Source: CAD feature listing. Evaluate the final solid. Frame: model axes, mm. Face numbers are marked on the shaded views. A direction names the side the tool comes from. Round coordinates to 2 decimals unless told otherwise and drop trailing zeros. Order: outer loops, then holes, each group sorted by start corner. A loop starts at its lowest first (then second) coordinate and runs counter-clockwise, first axis right, second up. Notation, with made-up numbers: (81, 83.25) -> (129, 83.25) arc R29 cw to (129, 110.25) -> close; hole circle Ø6 at (-18.75, 39). An arc over 180 degrees is marked (long way). Answer as CSV lines item,"result".
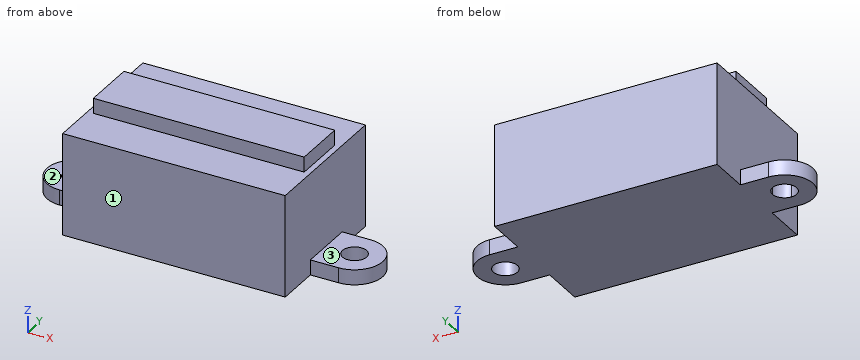
from build123d import *

# Parameters (mm, degrees)
F0_W     = 29.5
F0_H     = 18.9
F1_DEPTH = 13.5
F2_R     = 1.6
F3_DEPTH = 2
F4_W     = 27.95
F4_H     = 7.2
F5_DEPTH = 2


with BuildPart() as f1:
    # F0 (on Top) → F1 (new body)
    with BuildSketch(Plane.XY):
        with Locations((-2.3268059269, -8.9522809724)):
            Rectangle(F0_W, F0_H)
    extrude(amount=F1_DEPTH)

    # F2 (on face) → F3 (join)
    with BuildSketch(Plane(origin=(0, 0, 0), x_dir=(1, 0, 0), z_dir=(0, 0, -1))):
        with BuildLine():
            Line((-20.8268059269, 7.1262256302), (-20.8268059269, 4.9762256302))
            Line((-20.8268059269, 4.9762256302), (-17.0768059269, 4.9762256302))
            Line((-17.0768059269, 4.9762256302), (-17.0768059269, 12.4762256302))
            Line((-17.0768059269, 12.4762256302), (-20.8268059269, 12.4762256302))
            Line((-20.8268059269, 12.4762256302), (-20.8268059269, 10.3262256302))
            ThreePointArc((-20.8268059269, 10.3262256302), (-19.695435077, 9.8575964801), (-19.2268059269, 8.7262256302))
            ThreePointArc((-19.2268059269, 8.7262256302), (-19.695435077, 7.5948547803), (-20.8268059269, 7.1262256302))
        make_face()
        with BuildLine():
            ThreePointArc((-20.8268059269, 12.4762256302), (-24.5768059269, 8.7262256302), (-20.8268059269, 4.9762256302))
            Line((-20.8268059269, 4.9762256302), (-20.8268059269, 7.1262256302))
            ThreePointArc((-20.8268059269, 7.1262256302), (-22.4268059269, 8.7262256302), (-20.8268059269, 10.3262256302))
            Line((-20.8268059269, 10.3262256302), (-20.8268059269, 12.4762256302))
        make_face()
        with BuildLine():
            Line((12.4231940731, 12.4762256302), (12.4231940731, 4.9762256302))
            Line((12.4231940731, 4.9762256302), (16.1731940731, 4.9762256302))
            ThreePointArc((16.1731940731, 4.9762256302), (19.9231940731, 8.7262256302), (16.1731940731, 12.4762256302))
            Line((16.1731940731, 12.4762256302), (12.4231940731, 12.4762256302))
        make_face()
        with Locations((16.1731940731, 8.7262256302)):
            Circle(F2_R, mode=Mode.SUBTRACT)
    extrude(amount=-F3_DEPTH)

    # F4 (on face) → F5 (join)
    with BuildSketch(Plane.XY.offset(13.5)):
        with Locations((-2.3268059269, -8.9522809724)):
            Rectangle(F4_W, F4_H)
    extrude(amount=F5_DEPTH)


solid = f1.part
1. Section query A-A on x = 17. Return loops of the section in (y, z).
Results below:
outline,"(-12.38, 0) -> (-10.1, 0) -> (-10.1, 2) -> (-12.38, 2) -> close; (-7.36, 0) -> (-5.07, 0) -> (-5.07, 2) -> (-7.36, 2) -> close"
2. Section query D-D on y = -11. Return loops of the section in (x, z), and give its area (3 significant figures).
Results below:
outline,"(-23.81, 0) -> (19.16, 0) -> (19.16, 2) -> (12.42, 2) -> (12.42, 13.5) -> (11.65, 13.5) -> (11.65, 15.5) -> (-16.3, 15.5) -> (-16.3, 13.5) -> (-17.08, 13.5) -> (-17.08, 2) -> (-23.81, 2) -> close"
area,"481 mm2"
3. Pin query (flat end, axial travel): pin 1 (0.6 mm diameter, centred on y = -9, z = 14, fed in from +X); pin 2 (1 mm diameter, centred on x = 14.5, z = 1.5, fed in from +Y); pin 3 (3 mm diameter, centred on y = -7, z = 9.5, fed in from +X). Return the tip coordinate at first contact, or that it passes through.
Results below:
pin 1,"x = 11.65"
pin 2,"y = -4.98"
pin 3,"x = 12.42"
4. Reachability of the marked faces 1, 2 and 3 from +Z, -Z, +X, -X, +Y, -Y: full face, straight path, thin tool, end or side. Return the list, or none.
Results below:
face 1,"+Z, -Z, +X, -X, -Y"
face 2,"+Z, -X, +Y, -Y"
face 3,"+Z, +X, +Y, -Y"
5. Section query B-B on z = 10.75. Return loops of the section in (x, y).
Results below:
outline,"(-17.08, -18.4) -> (12.42, -18.4) -> (12.42, 0.5) -> (-17.08, 0.5) -> close"
6. Line query: L1, parallel to Z at x = 15, y = -10.25; L2, parallel to X at y = -0.25, z = 12.75; L3, parallel to Z at x = 5, y = -4.5. Output: solid intervals per line, ascending. Write a range as [from, to].
Results below:
L1,"[0, 2]"
L2,"[-17.08, 12.42]"
L3,"[0, 13.5]"
7. Section query C-C on x = 3.5. Return loops of the section in (y, z).
Results below:
outline,"(-18.4, 0) -> (0.5, 0) -> (0.5, 13.5) -> (-5.35, 13.5) -> (-5.35, 15.5) -> (-12.55, 15.5) -> (-12.55, 13.5) -> (-18.4, 13.5) -> close"
